```python
from build123d import *

# Parameters (mm, degrees)
F0_W      = 1219.2
F0_H      = 762
F1_DEPTH  = 406.4
F2_W      = 38.1
F2_H      = 38.1
F3_DEPTH  = 50.8
F4_W      = 1219.2
F4_H      = 406.4
F5_DEPTH  = 25.4
F7_DEPTH  = 6.35
F6_W      = 203.2
F6_H      = 660.4
F8_DEPTH  = 381
F9_W      = 254
F9_H      = 558.8
F10_DEPTH = 12.7
F9_W_2    = 3.175
F11_DEPTH = 25.4
F12_W     = 203.2
F12_H     = 19.05
F13_DEPTH = 355.6
F14_DEPTH = 50.8
F15_W     = 19.05
F15_H     = 19.05
F15_H_2   = 387.35
F15_W_2   = 31.75
F16_DEPTH = 50.8


with BuildPart() as f1:
    # F0 (on Front) → F1 (new body)
    with BuildSketch(Plane.XZ):
        Rectangle(F0_W, F0_H)
    extrude(amount=F1_DEPTH)

    # F2 (on face) → F3 (join)
    with BuildSketch(Plane(origin=(0, 0, -381), x_dir=(1, 0, 0), z_dir=(0, 0, -1))):
        with Locations((-590.55, 387.35)):
            Rectangle(F2_W, F2_H)
        with Locations((-590.55, 19.05)):
            Rectangle(F2_W, F2_H)
        with Locations((590.55, 387.35)):
            Rectangle(F2_W, F2_H)
        with Locations((590.55, 19.05)):
            Rectangle(F2_W, F2_H)
    extrude(amount=F3_DEPTH)

    # F4 (on face) → F5 (join)
    with BuildSketch(Plane.XY.offset(381)):
        with Locations((0, -203.2)):
            Rectangle(F4_W, F4_H)
        Polygon((-609.6, -406.4), (-609.6, 0), (-622.3, 0), (-622.3, -406.4), (-622.3, -431.8), (622.3, -431.8), (622.3, 0), (609.6, 0), (609.6, -406.4), align=None)
    extrude(amount=F5_DEPTH)

    # F6 (on face) → F7 (cut)
    with BuildSketch(Plane.XZ.offset(406.4)):
        Polygon((-101.6, 330.2), (-355.6, 330.2), (-355.6, -330.2), (0, -330.2), (0, 0), (0, 330.2), align=None)
        Polygon((355.6, 330.2), (0, 330.2), (0, 0), (0, -330.2), (355.6, -330.2), align=None)
    extrude(amount=-F7_DEPTH, mode=Mode.SUBTRACT)

    # F6 (on face) → F8 (cut)
    with BuildSketch(Plane.XZ.offset(406.4)):
        with Locations((-457.2, 0)):
            Rectangle(F6_W, F6_H)
        with Locations((457.2, 0)):
            Rectangle(F6_W, F6_H)
    extrude(amount=-F8_DEPTH, mode=Mode.SUBTRACT)

    # F9 (on face) → F10 (cut)
    with BuildSketch(Plane.XZ.offset(400.05)):
        with Locations((-177.8, 0)):
            Rectangle(F9_W, F9_H)
        with Locations((177.8, 0)):
            Rectangle(F9_W, F9_H)
    extrude(amount=-F10_DEPTH, mode=Mode.SUBTRACT)

    # F9 (on face) → F11 (cut)
    with BuildSketch(Plane.XZ.offset(400.05)):
        with Locations((1.5875, 0)):
            Rectangle(F9_W_2, F9_H)
        with Locations((-1.5875, 0)):
            Rectangle(F9_W_2, F9_H)
        Polygon((-3.175, -279.4), (-3.175, -330.2), (3.175, -330.2), (3.175, -279.4), (0, -279.4), align=None)
        Polygon((-3.175, 330.2), (-3.175, 279.4), (0, 279.4), (3.175, 279.4), (3.175, 330.2), align=None)
    extrude(amount=-F11_DEPTH, mode=Mode.SUBTRACT)

    # F12 (on face) → F13 (join)
    with BuildSketch(Plane.XZ.offset(25.4)):
        with Locations((-457.2, 119.507)):
            Rectangle(F12_W, F12_H)
        with Locations((-457.2, -100.711)):
            Rectangle(F12_W, F12_H)
        with Locations((457.2, -100.711)):
            Rectangle(F12_W, F12_H)
        with Locations((457.2, 119.507)):
            Rectangle(F12_W, F12_H)
    extrude(amount=F13_DEPTH)

    # F14 (cut): faces of the model
    f14_faces = [f1.faces().sort_by_distance(p)[0] for p in [
        (-590.55, -387.35, -431.8),
        (590.55, -387.35, -431.8),
        (590.55, -19.05, -431.8),
        (-590.55, -19.05, -431.8),
    ]]
    extrude(f14_faces, amount=-F14_DEPTH, mode=Mode.SUBTRACT)

    # F15 (on face) → F16 (join)
    with BuildSketch(Plane(origin=(0, 0, -381), x_dir=(1, 0, 0), z_dir=(0, 0, -1))):
        with Locations((-600.075, 396.875)):
            Rectangle(F15_W, F15_H)
        with Locations((-600.075, 193.675)):
            Rectangle(F15_W, F15_H_2)
        with Locations((600.075, 193.675)):
            Rectangle(F15_W, F15_H_2)
        with Locations((600.075, 396.875)):
            Rectangle(F15_W, F15_H)
        with Locations((574.675, 396.875)):
            Rectangle(F15_W_2, F15_H)
        with Locations((-574.675, 396.875)):
            Rectangle(F15_W_2, F15_H)
    extrude(amount=F16_DEPTH)


solid = f1.part
```
Source: CAD feature listing. Evaluate the final solid. Frame: model axes, mm. A direction names the side the tool comes from. Round coordinates to 2 decimals unless told otherwise and drop trailing zeros. Loops run counter-clockwise (first coordinate to the right, second up) from the corner with the lowest first, then second, coordinate; pieces in that order, holes last. Notation, with made-up numbers: M -36.75,15.5 L -28.75,15.5 A26 ccw -28.75,52.5 Z; hole C -34,31.5 d1. An arc over 180 degrees is marked long. Use a Markdown table: item, result. Add a question column.
1. Section query D-D on x = 67.5. Return the cut outline in (y, z), then the cut area to 3 significant figures.
2. Line query: line 1 (X direction, y = -35.5, z = 299); line 2 (Z direction, x = -424, y = -376); line 3 (X direction, y = -394, z = 243) (3 decimals). Output: solid intervals per line, ascending.
3. Section query A-A on x = 494. Return the cut outline in (y, z).
4. Section query C-C on y = -326. Give the number of separate pieces and of enclosed holes in the cut face, then the cut area to 3 significant figures.
5. Section query B-B on z = -171. Return the cut outline in (x, y) (3 decimals).
6. Contact query for flat-ended pins moving along their axis: P1, Ø6.5, axis at x = 139.5, y = -393.5, coming from the -Z side; P2, Ø3, axis at x = -137, z = -279, coming from the +Y side; P3, Ø8, axis at y = -151, z = 322.5, coming from the +X side; P4, Ø4, axis at x = -192.5, z = -192.5, coming from the -Y side. Output: stop coordinate, or through.
7. Reachability of faces 1 (the flat face through (574, -387.35, -406)), 2 (the flat face through (3, -406.4, 338)), 3 (the flat face through (456, -25.4, 11)) from +Z, -Z, +X, -X, +Y, -Y: full face, straight path, thin tool, end or side. Return the list, or none.
8. Mould query, pull axis X, two halves, no side actions, for faces 4 (the flat face through (176, -387.35, 4)), 5 (the flat face through (-459, -25.4, 231)), 6 (the flat face through (-9, 0, -7)), 7 (the flat face through (622.3, -219, 394)). Classes: pulls with the +X half, pulls with the -X half, needs draft (parallel to the pull), parting line crosses it, or undercut.
Reported:
| question | item | result |
|---|---|---|
| 1 | outline | M -431.8,381 L -406.4,381 L -406.4,330.2 L -400.05,330.2 L -400.05,279.4 L -387.35,279.4 L -387.35,-279.4 L -400.05,-279.4 L -400.05,-330.2 L -406.4,-330.2 L -406.4,-381 L 0,-381 L 0,406.4 L -431.8,406.4 Z |
| 1 | area | 309,000 mm² |
| 2 | line 1 | x = -609.6 to -558.8, -355.6 to 355.6, 558.8 to 609.6 |
| 2 | line 2 | z = -381 to -330.2, -110.24 to -91.19, 109.98 to 129.03, 330.2 to 406.4 |
| 2 | line 3 | x = -609.6 to -558.8, -355.6 to -304.8, -50.8 to -3.175, 3.175 to 50.8, 304.8 to 355.6, 558.8 to 609.6 |
| 3 | outline | M -431.8,381 L -406.4,381 L -406.4,330.2 L -25.4,330.2 L -25.4,129.03 L -381,129.03 L -381,109.98 L -25.4,109.98 L -25.4,-91.19 L -381,-91.19 L -381,-110.24 L -25.4,-110.24 L -25.4,-330.2 L -406.4,-330.2 L -406.4,-381 L 0,-381 L 0,406.4 L -431.8,406.4 Z |
| 4 | separate pieces | 1 |
| 4 | enclosed holes | 6 |
| 4 | area | 710,000 mm² |
| 5 | outline | M -609.6,-406.4 L -558.8,-406.4 L -558.8,-25.4 L -355.6,-25.4 L -355.6,-400.05 L -304.8,-400.05 L -304.8,-387.35 L -50.8,-387.35 L -50.8,-400.05 L -3.175,-400.05 L -3.175,-374.65 L 3.175,-374.65 L 3.175,-400.05 L 50.8,-400.05 L 50.8,-387.35 L 304.8,-387.35 L 304.8,-400.05 L 355.6,-400.05 L 355.6,-25.4 L 558.8,-25.4 L 558.8,-406.4 L 609.6,-406.4 L 609.6,0 L -609.6,0 Z |
| 6 | P1 | stops at z = -381 |
| 6 | P2 | stops at y = 0 |
| 6 | P3 | stops at x = 609.6 |
| 6 | P4 | stops at y = -387.35 |
| 7 | face 1 | -Z, +Y |
| 7 | face 2 | -Z, +X, -X, -Y |
| 7 | face 3 | -Y |
| 8 | face 4 | undercut |
| 8 | face 5 | undercut |
| 8 | face 6 | needs draft |
| 8 | face 7 | pulls with the +X half |
